Could you check a few things on this model? Use its own coordinates, in mm. A direction names the side the tool comes from. Give positions to 0.01 mm unless a question says otherwise; leave off trailing zeros. Order: outer loops, then holes, each group sorted by start corner. A loop starts at its lowest first (then second) coordinate and runs counter-clockwise, first axis right, second up. Notation, with made-up numbers: (-17, 18.5) -> (30, 18.5) arc R20 ccw to (30, 52.5) -> close; hole circle Ø4 at (-10.5, -28.75). An arc over 180 degrees is marked (long way). One line per item, written item: value.
```python
from build123d import *

# Parameters (mm, degrees)
SKETCH1_W           = 2.54
SKETCH1_H           = 1.524
BOSS_EXTRUDE1_DEPTH = 1.524


with BuildPart() as part:
    # Sketch1 → Boss-Extrude1 (new body)
    with BuildSketch(Plane.XY):
        with BuildLine():
            Line((109.975938606, -1.524), (107.383711033, -1.524))
            ThreePointArc((107.383711033, -1.524), (107.384970604, -2.46941588), (107.636449137, -3.380772737))
            ThreePointArc((107.636449137, -3.380772737), (107.992708895, -3.839670187), (108.528537329, -4.064160218))
            ThreePointArc((108.528537329, -4.064160218), (111.840473047, -3.687536777), (114.554773872, -1.752766908))
            ThreePointArc((114.554773872, -1.752766908), (114.642277966, -1.543971247), (114.595869935, -1.322388556))
            ThreePointArc((114.595869935, -1.322388556), (114.450356485, -0.762), (114.595869935, -0.201611444))
            ThreePointArc((114.595869935, -0.201611444), (114.642277966, 0.019971247), (114.554773872, 0.228766908))
            ThreePointArc((114.554773872, 0.228766908), (111.840473047, 2.163536777), (108.528537329, 2.540160218))
            ThreePointArc((108.528537329, 2.540160218), (107.992708895, 2.315670187), (107.636449137, 1.856772737))
            ThreePointArc((107.636449137, 1.856772737), (107.384970604, 0.94541588), (107.383711033, 0))
            Line((107.383711033, 0), (109.975938606, 0))
            Line((109.975938606, 0), (109.975938606, -1.524))
        make_face()
        with Locations((110.575658384, 1.133758123)):
            Rectangle(SKETCH1_W, SKETCH1_H, mode=Mode.SUBTRACT)
        with Locations((110.575658384, -2.657758123)):
            Rectangle(SKETCH1_W, SKETCH1_H, mode=Mode.SUBTRACT)
    extrude(amount=BOSS_EXTRUDE1_DEPTH)


solid = part.part
```
1) Suppose I cut it at B-B, the plane x = 111. Write out the boundary of the cut face in (y, z), then the cut area to 3 significant figures.
Answer below:
outline: (-3.95, 0) -> (-3.42, 0) -> (-3.42, 1.52) -> (-3.95, 1.52) -> close; (-1.9, 0) -> (0.37, 0) -> (0.37, 1.52) -> (-1.9, 1.52) -> close; (1.9, 0) -> (2.42, 0) -> (2.42, 1.52) -> (1.9, 1.52) -> close
area: 5.06 mm2
2) Suppose I cut it at A-A, the plane z = 0.75. Write out the boundary of the cut face in (x, y).
Answer below:
outline: (107.38, -1.52) arc R3.54 ccw to (107.64, -3.38) arc R1.14 ccw to (108.53, -4.06) arc R6.66 ccw to (114.55, -1.75) arc R0.38 ccw to (114.6, -1.32) arc R1.15 cw to (114.6, -0.2) arc R0.38 ccw to (114.55, 0.23) arc R6.66 ccw to (108.53, 2.54) arc R1.14 ccw to (107.64, 1.86) arc R3.54 ccw to (107.38, 0) -> (109.98, 0) -> (109.98, -1.52) -> close; hole (109.31, -3.42) -> (111.85, -3.42) -> (111.85, -1.9) -> (109.31, -1.9) -> close; hole (109.31, 0.37) -> (111.85, 0.37) -> (111.85, 1.9) -> (109.31, 1.9) -> close
3) We'd pull the mould along Y, two halves only. Please class faces 1 (the flat face through (111.846, -3, 1)), 2 (the flat face through (109.306, -3, 1)), 3 (the flat face through (111, -1, 1.524)), 4 (the cylindrical face through (111.796, -3.704, 0.751)): +Y half, -Y half, draft (parallel to the pull), parting line (faces both ways), or undercut.
Answer below:
face 1: undercut
face 2: undercut
face 3: draft
face 4: -Y half
4) For P1, Ø0.5, axis at x = 110, z = 0.5, coming from the -Y side; P2, Ø0.8, axis at x = 111, z = 0.5, coming from the +Y side; P3, Ø1, axis at x = 110, y = -2.5, coming from the +Z side; P4, Ø0.8, axis at y = -2.5, z = 0.5, coming from the -X side, each with a flat end and sliding along its axis, tell me the tip position at first contact or that it passes through.
Answer below:
P1: stops at y = -4.12
P2: stops at y = 2.51
P3: passes through
P4: stops at x = 107.35
5) Suppose I cut it at C-C, the plane y = -3. Write out the boundary of the cut face in (x, z).
Answer below:
outline: (107.5, 0) -> (109.31, 0) -> (109.31, 1.52) -> (107.5, 1.52) -> close; (111.85, 0) -> (113.17, 0) -> (113.17, 1.52) -> (111.85, 1.52) -> close
6) If I drill on line 1 along Y through (x, z) = (110.75, 0.1); line 2 along Y through (x, z) = (108.5, 1); line 3 along X through (y, z) = (-3.25, 0.25), over which ranges is the centre line in solid material (lowest first)?
Answer below:
line 1: y = -4 to -3.42, -1.9 to 0.37, 1.9 to 2.48
line 2: y = -4.06 to -1.52, 0 to 2.54
line 3: x = 107.58 to 109.31, 111.85 to 112.76
7) For faces 5 (the flat face through (111, 1.896, 1)), 6 (the flat face through (109.976, -1, 1)), 7 (the cylindrical face through (114.45, -0.77, 0.75)), which set-ups out of +Z, -Z, +X, -X, +Y, -Y let a thin tool reach every point of the face, with its end or its side?
Answer below:
face 5: +Z, -Z
face 6: +Z, -Z, -X
face 7: +Z, -Z, +X
8) Suppose I cut it at D-D, the plane y = -2.25. Write out the boundary of the cut face in (x, z).
Answer below:
outline: (107.36, 0) -> (109.31, 0) -> (109.31, 1.52) -> (107.36, 1.52) -> close; (111.85, 0) -> (114.09, 0) -> (114.09, 1.52) -> (111.85, 1.52) -> close
